Can you work these out from the model? Positions are in its coordinate system, mm. A direction names the side the tool comes from. Give positions to 0.01 mm unless a question says otherwise; leave off trailing zeros. Loops run counter-clockwise (first coordinate to the right, second up) from the corner with the lowest first, then second, coordinate; pieces in that order, holes last. Notation, with made-up numbers: (-28, 57.25) - (27, 57.25) arc R34 ccw to (27, 87.25) - close; hole circle Ø1 at (20, -10.5). An arc over 180 degrees is marked (long way). Answer as a JSON object with one key per item and string values.
```python
from build123d import *

# Parameters (mm, degrees)
SKETCH1_W               = 63.5
SKETCH1_H               = 10.16
BOSS_EXTRUDE1_DEPTH     = 51
SKETCH2_R               = 1.0922
CUT_EXTRUDE1_DEPTH      = 10
CUT_EXTRUDE2_DEPTH      = 83.076035479
CUT_EXTRUDE2_DEPTH_BACK = 83.076035479
SKETCH3_W               = 8
SKETCH3_H               = 47.710038991
SKETCH3_H_2             = 48.198954848
SKETCH5_W               = 33
SKETCH5_H               = 10.16
SKETCH5_R               = 1.363261963
SKETCH5_W_2             = 27.5
SKETCH5_R_2             = 1.386126721
BOSS_EXTRUDE2_DEPTH     = 6
CHAMFER2_SIZE           = 15
CUT_EXTRUDE3_DEPTH      = 98.945013145
CUT_EXTRUDE3_DEPTH_BACK = 98.945013145
SKETCH6_W               = 9.1
SKETCH6_H               = 10.9
SKETCH6_R               = 1.849544376
SKETCH6_R_2             = 1.82922697
SKETCH7_W               = 9.1
SKETCH7_H               = 10.9
BOSS_EXTRUDE3_DEPTH     = 1.66
SKETCH8_W               = 1.75
SKETCH8_H               = 7.5
BOSS_EXTRUDE4_DEPTH     = 3


with BuildPart() as part:
    # Sketch1 → Boss-Extrude1 (new body)
    with BuildSketch(Plane(origin=(0, 0, 0), x_dir=(1, 0, 0), z_dir=(0, 1, 0))):
        with Locations((31.75, 5.08)):
            Rectangle(SKETCH1_W, SKETCH1_H)
    extrude(amount=BOSS_EXTRUDE1_DEPTH)

    # Sketch2 → Cut-Extrude1 (cut)
    with BuildSketch(Plane(origin=(0, 0, 0), x_dir=(-1, 0, 0), z_dir=(0, -1, 0))):
        with Locations(Location((-59.75, 2.5, 0), (0, 0, 90))):
            Circle(SKETCH2_R)
        with Locations(Location((-3.75, 2.5, 0), (0, 0, 90))):
            Circle(SKETCH2_R)
    extrude(amount=-CUT_EXTRUDE1_DEPTH, mode=Mode.SUBTRACT)

    # Sketch3 → Cut-Extrude2 (cut, two sides: drawn at the far end of the back side and taken through both)
    with BuildSketch(Plane.XY.offset(-CUT_EXTRUDE2_DEPTH_BACK)):
        with Locations((4, 29.452019142)):
            Rectangle(SKETCH3_W, SKETCH3_H)
        with Locations((59.5, 28.066757549)):
            Rectangle(SKETCH3_W, SKETCH3_H_2)
    extrude(amount=CUT_EXTRUDE2_DEPTH + CUT_EXTRUDE2_DEPTH_BACK, mode=Mode.SUBTRACT)

    # Sketch5 → Boss-Extrude2 (add)
    # profile 1 of 2: a face of its own
    with BuildSketch(Plane(origin=(0, 51, 0), x_dir=(1, 0, 0), z_dir=(0, 1, 0))):
        with Locations((-8.5, 5.08)):
            Rectangle(SKETCH5_W, SKETCH5_H)
        with Locations(Location((-20, 5.16, 0), (0, 0, 270))):
            Circle(SKETCH5_R, mode=Mode.SUBTRACT)
    # profile 2 of 2: a face of its own
    with BuildSketch(Plane(origin=(0, 51, 0), x_dir=(1, 0, 0), z_dir=(0, 1, 0))):
        with Locations((69.25, 5.08)):
            Rectangle(SKETCH5_W_2, SKETCH5_H)
        with Locations(Location((78, 5.16, 0), (0, 0, 270))):
            Circle(SKETCH5_R_2, mode=Mode.SUBTRACT)
    extrude(amount=-BOSS_EXTRUDE2_DEPTH)

    # Chamfer2
    chamfer2_edges = [part.edges().sort_by_distance(p)[0] for p in [
        (8, 45, -5.08),
        (55.5, 45, -5.08),
    ]]
    chamfer(chamfer2_edges, length=CHAMFER2_SIZE)

    # Sketch6 → Cut-Extrude3 (cut, two sides: drawn at the far end of the back side and taken through both)
    with BuildSketch(Plane.XY.offset(-CUT_EXTRUDE3_DEPTH_BACK)):
        with Locations((31.75, 23.45)):
            Rectangle(SKETCH6_W, SKETCH6_H)
        Polygon((27.2, 18), (17, 18), (17, 15.25), (17, 11.5), (17, 7.75), (17, 5), (46.5, 5), (46.5, 7.75), (46.5, 11.5), (46.5, 15.25), (46.5, 18), (36.3, 18), align=None)
        with BuildLine():
            Line((17, 11.5), (17, 15.25))
            Line((17, 15.25), (15.25, 15.25))
            Line((15.25, 15.25), (15.25, 14.672144385))
            ThreePointArc((15.25, 14.672144385), (16.533481384, 13.311422093), (17, 11.5))
        make_face()
        with BuildLine():
            Line((17, 7.75), (17, 11.5))
            ThreePointArc((17, 11.5), (16.533481384, 9.688577907), (15.25, 8.327855615))
            Line((15.25, 8.327855615), (15.25, 7.75))
            Line((15.25, 7.75), (17, 7.75))
        make_face()
        with Locations((13.25, 11.5)):
            Circle(SKETCH6_R)
        with Locations((50.25, 11.5)):
            Circle(SKETCH6_R_2)
        with BuildLine():
            Line((48.25, 15.25), (46.5, 15.25))
            Line((46.5, 15.25), (46.5, 11.5))
            ThreePointArc((46.5, 11.5), (46.966518616, 13.311422093), (48.25, 14.672144385))
            Line((48.25, 14.672144385), (48.25, 15.25))
        make_face()
        with BuildLine():
            ThreePointArc((48.25, 8.327855615), (46.966518616, 9.688577907), (46.5, 11.5))
            Line((46.5, 11.5), (46.5, 7.75))
            Line((46.5, 7.75), (48.25, 7.75))
            Line((48.25, 7.75), (48.25, 8.327855615))
        make_face()
    extrude(amount=CUT_EXTRUDE3_DEPTH + CUT_EXTRUDE3_DEPTH_BACK, mode=Mode.SUBTRACT)

    # Sketch7 → Boss-Extrude3 (add)
    with BuildSketch(Plane(origin=(0, 0, -10.16), x_dir=(-1, 0, 0), z_dir=(0, 0, -1))):
        with Locations((-31.75, 23.45)):
            Rectangle(SKETCH7_W, SKETCH7_H)
    extrude(amount=-BOSS_EXTRUDE3_DEPTH)

    # Sketch8 → Boss-Extrude4 (add)
    with BuildSketch(Plane(origin=(0, 0, -10.16), x_dir=(-1, 0, 0), z_dir=(0, 0, -1))):
        with Locations((-47.375, 11.5)):
            Rectangle(SKETCH8_W, SKETCH8_H)
        with Locations((-16.125, 11.5)):
            Rectangle(SKETCH8_W, SKETCH8_H)
    extrude(amount=-BOSS_EXTRUDE4_DEPTH)


solid = part.part
```
1) I'm going to push flat-ended pins straight in: P1, Ø3, axis at y = 1.5, z = -4.5, coming from the +X side; P2, Ø1.5, axis at y = 14, z = -2.5, coming from the -X side; P3, Ø0.9, axis at x = 47, y = 10.5, coming from the +Z side; P4, Ø2, axis at x = 59.75, z = -2.5, coming from the -Y side. Where does each tip first touch, or does it pass through?
Check sheet entries:
{"P1": "x = 63.5", "P2": "x = 8", "P3": "z = 0", "P4": "y = 33.25"}
2) Imagine slicing it at D-D on z = -5.16. Give the number of separate pieces and of enclosed holes in the cut face, and give its area (3 significant figures).
Check sheet entries:
{"separate pieces": "3", "enclosed holes": "3", "area": "2,540 mm2"}
3) Imagine slicing it at A-A on x = 78. Write out the boundary of the cut face in (y, z).
Check sheet entries:
{"outline": "(45, -10.16) - (51, -10.16) - (51, -6.55) - (45, -6.55) - close; (45, -3.77) - (51, -3.77) - (51, 0) - (45, 0) - close"}
4) If we mould it in two halves opening along Y, with no side actions, what happens to faces 1 (the flat face through (30, 32, -10.16)), 2 (the flat face through (-16, 45, -5)), 3 (the cylindrical face through (51.94, 10.8, -5.15))? For each: released by +Y, released by -Y, zero draft, split by the parting line, or undercut.
Check sheet entries:
{"face 1": "zero draft", "face 2": "released by -Y", "face 3": "undercut"}
5) Which directions (+Z, -Z, +X, -X, +Y, -Y) give clear straight access to the entire face, cutting with the end or side of a thin tool? Please do faces 4 (the flat face through (36.3, 23, -4)), 5 (the flat face through (55.5, 17, -5)), 6 (the flat face through (8, 18, -5)).
Check sheet entries:
{"face 4": "+Z", "face 5": "+Z, -Z, +X", "face 6": "+Z, -Z, -X"}
6) Imagine slicing it at B-B on y = 22. Write out the boundary of the cut face in (x, z), and give its area (3 significant figures).
Check sheet entries:
{"outline": "(8, -10.16) - (55.5, -10.16) - (55.5, 0) - (36.3, 0) - (36.3, -8.5) - (27.2, -8.5) - (27.2, 0) - (8, 0) - close", "area": "405 mm2"}
7) I need wall thicknesses on L1, parallel to X at y = 49.25, z = -5.16; L2, parallel to X at y = 3.4, z = -2.5; L3, parallel to X at y = 11.5, z = -5.5. Which ranges of each line are inside material? Lowest first, please.
Check sheet entries:
{"L1": "-25 to -21.36, -18.64 to 76.61, 79.39 to 83", "L2": "0 to 2.66, 4.84 to 58.66, 60.84 to 63.5", "L3": "8 to 11.4, 15.1 to 17, 46.5 to 48.42, 52.08 to 55.5"}
8) Imagine slicing it at C-C on x = 59.75. Write out the boundary of the cut face in (y, z), and give its area (3 significant figures).
Check sheet entries:
{"outline": "(0, -10.16) - (3.97, -10.16) - (3.97, -3.59) - (0, -3.59) - close; (0, -1.41) - (3.97, -1.41) - (3.97, 0) - (0, 0) - close; (34.25, -10.16) - (51, -10.16) - (51, 0) - (34.25, 0) - close", "area": "202 mm2"}
